Source: CAD feature listing. Evaluate the final solid. Frame: model axes, mm. A direction names the side the tool comes from. Give positions to 0.01 mm unless a question says otherwise; leave off trailing zeros. Order: outer loops, then holes, each group sorted by start corner. A loop starts at its lowest first (then second) coordinate and runs counter-clockwise, first axis right, second up. Notation, with made-up numbers: (46, 33) - (95, 33) arc R5 cw to (95, 42) - close; hole circle Ø4 at (25, 26). An arc over 180 degrees is marked (long way). Answer as CSV lines item,"result".
```python
from build123d import *

# Parameters (mm, degrees)
SKETCH1_W              = 46
SKETCH1_H              = 38
BOSS_EXTRUDE1_DEPTH    = 15
M10X1_0_TAPPED_HOLE1_D = 9
SKETCH7_R              = 7.95
CUT_EXTRUDE1_DEPTH     = 62.522353661
SKETCH17_W             = 38
SKETCH17_H             = 5
BOSS_EXTRUDE2_DEPTH    = 10
SKETCH18_W             = 38
SKETCH18_H             = 5
BOSS_EXTRUDE3_DEPTH    = 10
SKETCH24_W             = 18.029816061
SKETCH24_H             = 38
BOSS_EXTRUDE4_DEPTH    = 6


with BuildPart() as part:
    # Sketch1 → Boss-Extrude1 (new body)
    with BuildSketch(Plane(origin=(0, 0, 0), x_dir=(1, 0, 0), z_dir=(0, 1, 0))):
        with Locations((23, 19)):
            Rectangle(SKETCH1_W, SKETCH1_H)
    extrude(amount=BOSS_EXTRUDE1_DEPTH)

    # M10x1.0 Tapped Hole1 (through all)
    with Locations(Plane(origin=(0, 15, 0), x_dir=(1, 0, 0), z_dir=(0, 1, 0))):
        with Locations((7.5, 29), (38.5, 29), (38.5, 9), (7.5, 9)):
            Hole(M10X1_0_TAPPED_HOLE1_D / 2)

    # Sketch7 → Cut-Extrude1 (cut, through all)
    with BuildSketch(Plane.XY):
        with Locations((23, 15)):
            Circle(SKETCH7_R)
    extrude(amount=-CUT_EXTRUDE1_DEPTH, mode=Mode.SUBTRACT)

    # Sketch17 → Boss-Extrude2 (add)
    with BuildSketch(Plane(origin=(46, 0, 0), x_dir=(0, 0, -1), z_dir=(1, 0, 0))):
        with Locations((19, 2.5)):
            Rectangle(SKETCH17_W, SKETCH17_H)
    extrude(amount=BOSS_EXTRUDE2_DEPTH)

    # Sketch18 → Boss-Extrude3 (add)
    with BuildSketch(Plane.ZY):
        with Locations((-19, 2.5)):
            Rectangle(SKETCH18_W, SKETCH18_H)
    extrude(amount=BOSS_EXTRUDE3_DEPTH)

    # Sketch24 → Boss-Extrude4 (add)
    with BuildSketch(Plane(origin=(0, 9.45, 0), x_dir=(1, 0, 0), z_dir=(0, 1, 0))):
        with Locations((23.165854861, 19)):
            Rectangle(SKETCH24_W, SKETCH24_H)
    extrude(amount=-BOSS_EXTRUDE4_DEPTH)


solid = part.part
```
(1) Contact query for flat-ended pins moving along their axis: pin 1 (1 mm diameter, centred on x = 48, z = -12, fed in from +Y); pin 2 (3 mm diameter, centred on y = 9, z = -21.5, fed in from +X); pin 3 (5.5 mm diameter, centred on x = 21, z = -19.5, fed in from +Y). Output: stop coordinate, or through.
Completed:
pin 1,"y = 5"
pin 2,"x = 46"
pin 3,"y = 9.45"
(2) Cut plane D-D (z = -34.5). Return loops of the section in (x, y).
Completed:
outline,"(-10, 0) - (56, 0) - (56, 5) - (46, 5) - (46, 15) - (30.95, 15) arc R7.95 cw to (28.69, 9.45) - (17.31, 9.45) arc R7.95 cw to (15.05, 15) - (0, 15) - (0, 5) - (-10, 5) - close"
(3) Access query for faces 1 (the flat face through (56, 3, -19)), 2 (the cylindrical face through (30.348, 11.964, -18.734)), 3 (the flat face through (23, 0, -19)), 4 (the flat face through (46, 10, -19)), 5 (the flat face through (-5, 5, -19)). Directions: +Z, -Z, +X, -X, +Y, -Y. A direction counts if a zero-diameter tool reaches every point of the face in a straight line with its end or side. Return the directions, or none.
Completed:
face 1,"+Z, -Z, +X, +Y, -Y"
face 2,"+Z, -Z, +Y"
face 3,"+Z, -Z, +X, -X, -Y"
face 4,"+Z, -Z, +X, +Y"
face 5,"+Z, -Z, -X, +Y"
(4) Cut plane C-C (y = 2). Return loops of the section in (x, z).
Completed:
outline,"(-10, -38) - (56, -38) - (56, 0) - (-10, 0) - close; hole circle Ø9 at (7.5, -29); hole circle Ø9 at (7.5, -9); hole circle Ø9 at (38.5, -29); hole circle Ø9 at (38.5, -9)"
(5) Ray query, line 1 (Z direction, x = 7.5, y = 7.5); line 2 (X direction, y = 4.5, z = -28); line 3 (X direction, y = 14.5, z = -33). Return the intervals inside material, ascending. Write a range as from..to.
Completed:
line 1,"-38..-33.5, -24.5..-13.5, -4.5..0"
line 2,"-10..3.11, 11.89..34.11, 42.89..56"
line 3,"0..5.44, 9.56..15.07, 30.93..36.44, 40.56..46"
(6) Mould query, pull axis Z, two halves, no side actions, for faces 6 (the flat face through (23, 6, -38)), 7 (the flat face through (51, 5, -19)), 8 (the cylindrical face through (3.208, 7.395, -10.352)), 9 (the cylindrical face through (5.42, 7.4, -25.01)). Classes: released by +Z, released by -Z, zero draft, split by the parting line, or undercut.
Completed:
face 6,"released by -Z"
face 7,"zero draft"
face 8,"undercut"
face 9,"undercut"
(7) Cut plane A-A (x = 7.5). Return loops of the section in (y, z).
Completed:
outline,"(0, -38) - (15, -38) - (15, -33.5) - (0, -33.5) - close; (0, -24.5) - (15, -24.5) - (15, -13.5) - (0, -13.5) - close; (0, -4.5) - (15, -4.5) - (15, 0) - (0, 0) - close"
(8) Cut plane B-B (z = -9). Return loops of the section in (x, y).
Completed:
outline,"(-10, 0) - (3, 0) - (3, 15) - (0, 15) - (0, 5) - (-10, 5) - close; (12, 0) - (34, 0) - (34, 15) - (30.95, 15) arc R7.95 cw to (28.69, 9.45) - (17.31, 9.45) arc R7.95 cw to (15.05, 15) - (12, 15) - close; (43, 0) - (56, 0) - (56, 5) - (46, 5) - (46, 15) - (43, 15) - close"
